from build123d import *

# Parameters (mm, degrees)
F0_R     = 22.5
F0_R_2   = 5.5
F1_DEPTH = 8
F2_R     = 22.5
F2_R_2   = 15.5
F3_DEPTH = 3
F4_SIZE  = 0.5
F5_SIZE  = 0.5


with BuildPart() as f1:
    # F0 (on Front) → F1 (new body)
    with BuildSketch(Plane.XZ):
        Circle(F0_R)
        Circle(F0_R_2, mode=Mode.SUBTRACT)
    extrude(amount=F1_DEPTH)

    # F2 (on face) → F3 (cut)
    with BuildSketch(Plane.XZ.offset(8)):
        Circle(F2_R)
        Circle(F2_R_2, mode=Mode.SUBTRACT)
    extrude(amount=-F3_DEPTH, mode=Mode.SUBTRACT)

    # F4
    f4_edges = [f1.edges().sort_by_distance(p)[0] for p in [
        (-22.5, 0, 0),
        (-22.5, -5, 0),
        (-15.5, -8, 0),
    ]]
    chamfer(f4_edges, length=F4_SIZE)

    # F5
    f5_edges = [f1.edges().sort_by_distance(p)[0] for p in [
        (-5.5, -8, 0),
        (-5.5, 0, 0),
    ]]
    chamfer(f5_edges, length=F5_SIZE)


solid = f1.part
Can you work these out from the model? Positions are in its coordinate system, mm. A direction names the side the tool comes from. Coordinates: 2 decimals unless noted, no trailing zeros. Write each loop counter-clockwise with the first axis right and the second up, starting at its lowest first coordinate (ties: lowest second). Pieces come first, ordered by that corner, then holes. Notation, with made-up numbers: (-11, 32) - (27, 32) arc R19 cw to (27, 64) - close; hole circle Ø4 at (-18.75, 34.5). An arc over 180 degrees is marked (long way). Return JSON: item names as keys, results as strings. Group by question number.
Item 1: I'm going to push flat-ended pins straight in: pin 1 Ø10 at (x, z) = (1.5, 17.5) entering from +Y; pin 2 Ø4 at (y, z) = (-2.5, 3.5) entering from -X; pin 3 Ø6.5 at (x, z) = (0, 0) entering from +Y. Where does each tip first touch, or does it pass through?
Item 2: If we section it at A-A (x = 0): Write out the boundary of the cut face in (y, z), then the cut area to 3 significant figures.
Item 3: Which directions (+Z, -Z, +X, -X, +Y, -Y) give clear straight access to the entire face, cutting with the end or side of a thin tool? Please do faces 4 (the face through (5, -5, 15)), 5 (the face through (6.5, -8, 0.2)).
Item 4: Please list where these lines run through material, in increasing order: probe 1 along Z at (x, y) = (0, -3); probe 2 along Z at (x, y) = (0, -5.75); probe 3 along X at (y, z) = (-1, -4.5).
Item 5: We'd pull the mould along X, two halves only. Please class faces 1 (the face through (-1.19, -3.95, -5.37)), 2 (the face through (5, 0, -5)), 3 (the face through (-2.018, -6.268, 15.368)): pulls with the +X half, pulls with the -X half, needs draft (parallel to the pull), parting line crosses it, or undercut.
Item 6: If we section it at C-C (y = -1.25): Write out the boundary of the cut face in (x, z), then the cut area to 3 significant figures.
Item 7: If we section it at B-B (z = 0): Write out the boundary of the cut face in (x, y), then the cut area to 3 significant figures.
Return value:
{
 "1": {"pin 1": "stops at y = 0", "pin 2": "stops at x = -22.45", "pin 3": "passes through"},
 "2": {"outline": "(-8, -15) - (-7.5, -15.5) - (-5, -15.5) - (-5, -22) - (-4.5, -22.5) - (-0.5, -22.5) - (0, -22) - (0, -6) - (-0.5, -5.5) - (-7.5, -5.5) - (-8, -6) - close; (-8, 6) - (-7.5, 5.5) - (-0.5, 5.5) - (0, 6) - (0, 22) - (-0.5, 22.5) - (-4.5, 22.5) - (-5, 22) - (-5, 15.5) - (-7.5, 15.5) - (-8, 15) - close", "area": "229 mm^2"},
 "3": {"face 4": "-Y", "face 5": "+Z, -Z, +X, -X, -Y"},
 "4": {"probe 1": "z = -22.5 to -5.5, 5.5 to 22.5", "probe 2": "z = -15.5 to -5.5, 5.5 to 15.5", "probe 3": "x = -22.05 to -3.16, 3.16 to 22.05"},
 "5": {"face 1": "undercut", "face 2": "needs draft", "face 3": "parting line crosses it"},
 "6": {"outline": "circle Ø45 at (0, 0); hole circle Ø11 at (0, 0)", "area": "1,500 mm^2"},
 "7": {"outline": "(-22.5, -4.5) - (-22, -5) - (-15.5, -5) - (-15.5, -7.5) - (-15, -8) - (-6, -8) - (-5.5, -7.5) - (-5.5, -0.5) - (-6, 0) - (-22, 0) - (-22.5, -0.5) - close; (5.5, -7.5) - (6, -8) - (15, -8) - (15.5, -7.5) - (15.5, -5) - (22, -5) - (22.5, -4.5) - (22.5, -0.5) - (22, 0) - (6, 0) - (5.5, -0.5) - close", "area": "229 mm^2"}
}
